Input: dimensioned drawing with shaded views. Units: mm. Origin: part minimum x, y, z. A direction names the side the tool comes from. Give positions to 0.01 mm unless a question says otherwise; leave off trailing zeros. Order: outer loops, then holes, each group sorted by start corner. A loop starts at its lowest first (then second) coordinate and runs counter-clockwise, first axis right, second up.
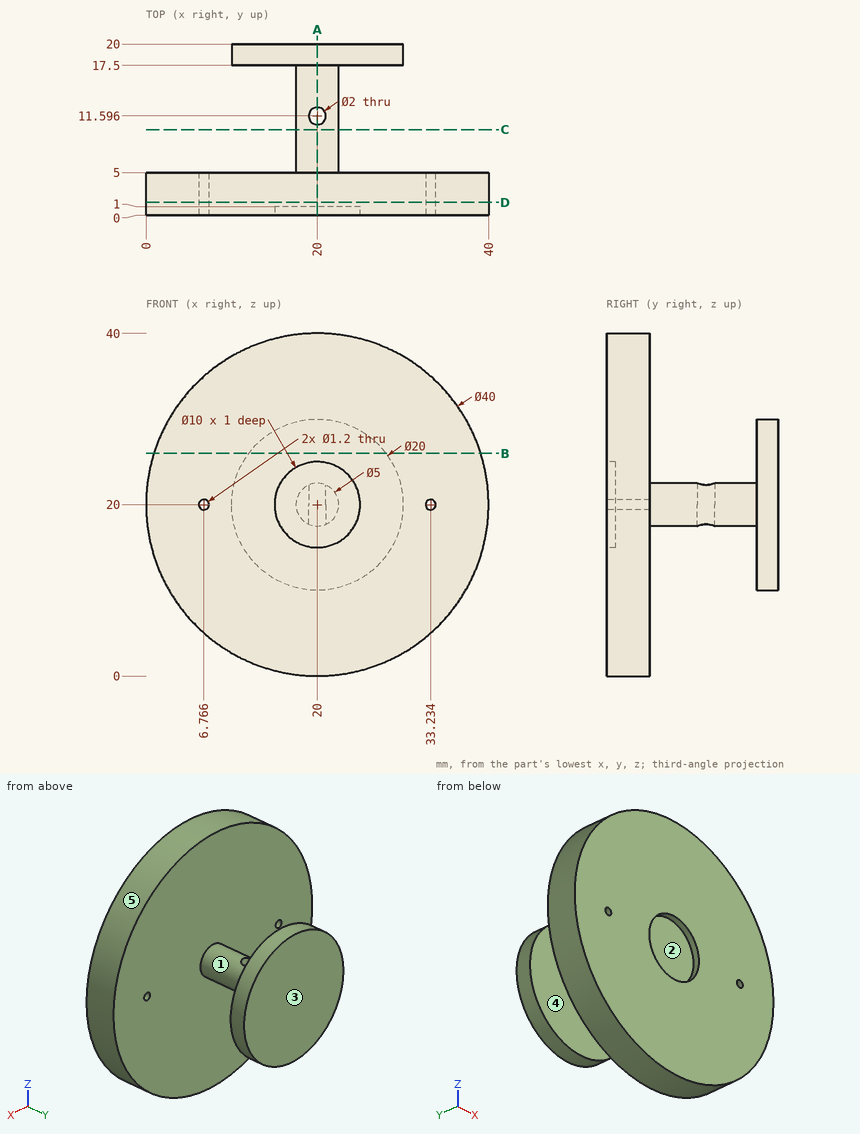
1) Reachability of the marked faces 4 and 5 from +Z, -Z, +X, -X, +Y, -Y: full face, straight path, thin tool, end or side. Return the list, or none.
Report:
face 4: none
face 5: +Y, -Y
2) Section query D-D, the plane y = 1.5. Return the cut outline in (x, z).
Report:
outline: circle Ø40 at (20, 20); hole circle Ø1.2 at (6.77, 20); hole circle Ø1.2 at (33.23, 20)
3) Material intervals for L1, parallel to Y at x = 16, z = 22.5; L2, parallel to Y at x = 13.5, z = 14; L3, parallel to Z at x = 20, y = 0.75, sorted ascending.
Report:
L1: y = 1 to 5, 17.5 to 20
L2: y = 0 to 5, 17.5 to 20
L3: z = 0 to 15, 25 to 40
4) Section query C-C, the plane y = 10. Return the cut outline in (x, z), and give its area (3 significant figures).
Report:
outline: circle Ø5 at (20, 20)
area: 19.6 mm2
5) Section query A-A, the plane x = 20. Return the cut outline in (y, z).
Report:
outline: (0, 0) - (5, 0) - (5, 17.5) - (10.6, 17.5) - (10.6, 22.5) - (5, 22.5) - (5, 40) - (0, 40) - (0, 25) - (1, 25) - (1, 15) - (0, 15) - close; (12.6, 17.5) - (17.5, 17.5) - (17.5, 10) - (20, 10) - (20, 30) - (17.5, 30) - (17.5, 22.5) - (12.6, 22.5) - close
6) Draft query along Z for the marked faces 1, 2 and 3. Return one class per face: +Z half, -Z half, draft (parallel to the pull), parting line (faces both ways), or undercut.
Report:
face 1: parting line
face 2: undercut
face 3: draft
7) Section query B-B, the plane z = 26. Return the cut outline in (x, y), and give its area (3 significant figures).
Report:
outline: (0.92, 0) - (39.08, 0) - (39.08, 5) - (0.92, 5) - close; (12, 17.5) - (28, 17.5) - (28, 20) - (12, 20) - close
area: 231 mm2
8) Pin query (flat end, axial travel): pin 1 (2.5 mm diameter, centred on x = 20, y = 11.6, fed in from +Z); pin 2 (3 mm diameter, centred on x = 22, z = 18.5, fed in from -Y); pin 3 (1.4 mm diameter, centred on x = 6.77, z = 20, fed in from +Y); pin 4 (4 mm diameter, centred on x = 24.5, z = 7.5, fed in from -Y). Return the tip coordinate at first contact, or that it passes through.
Report:
pin 1: stops at z = 22.5
pin 2: stops at y = 1
pin 3: stops at y = 5
pin 4: stops at y = 0
